Design review of the part built by this model. Coordinates are the model's own, in mm. A direction names the side the tool comes from. Give positions to 0.01 mm unless a question says otherwise; leave off trailing zeros. Loops run counter-clockwise (first coordinate to the right, second up) from the corner with the lowest first, then second, coordinate; pieces in that order, holes last. Notation, with made-up numbers: M 65.5,61 L 118.5,61 A15 cw 118.5,78 Z; hole C -19,56.5 d10. An arc over 180 degrees is marked long. Use CSV: the item, a comma, the result in double quotes.
from build123d import *

# Parameters (mm, degrees)
RESSALTO_EXTRUS_O2_DEPTH  = 19
ESBO_O2_R                 = 2
RESSALTO_EXTRUS_O3_DEPTH  = 5
FILETE1_R                 = 3
ESBO_O3_R                 = 4
RESSALTO_EXTRUS_O4_DEPTH  = 17
RESSALTO_EXTRUS_O6_START  = 10
ESBO_O4_R                 = 4
RESSALTO_EXTRUS_O6_DEPTH  = 10
ESBO_O5_R                 = 4
RESSALTO_EXTRUS_O7_DEPTH  = 10
RESSALTO_EXTRUS_O10_DEPTH = 27
FILETE2_R                 = 10
ESBO_O8_R                 = 5
ESBO_O8_R_2               = 4
RESSALTO_EXTRUS_O11_DEPTH = 2


with BuildPart() as part:
    # Esbo_o1 → Ressalto-extrus_o2 (new body)
    with BuildSketch(Plane.XY):
        with BuildLine():
            Line((-5.964101615, -2), (-3.464101615, -2))
            ThreePointArc((-3.464101615, -2), (4, 0), (-3.464101615, 2))
            Line((-3.464101615, 2), (-5.964101615, 2))
            Line((-5.964101615, 2), (-5.964101615, -2))
        make_face()
    extrude(amount=RESSALTO_EXTRUS_O2_DEPTH)

    # Esbo_o2 → Ressalto-extrus_o3 (add)
    with BuildSketch(Plane.XY.offset(19)):
        with BuildLine():
            Line((-20, -5), (-8.660254038, -5))
            ThreePointArc((-8.660254038, -5), (10, 0), (-8.660254038, 5))
            Line((-8.660254038, 5), (-20, 5))
            Line((-20, 5), (-20, -5))
        make_face()
        with Locations((-15, 0)):
            Circle(ESBO_O2_R, mode=Mode.SUBTRACT)
    extrude(amount=RESSALTO_EXTRUS_O3_DEPTH)

    # Filete1
    filete1_edges = [part.edges().sort_by_distance(p)[0] for p in [
        (-20, 5, 21.5),
        (-20, -5, 21.5),
    ]]
    fillet(filete1_edges, radius=FILETE1_R)

    # Esbo_o3 → Ressalto-extrus_o4 (add)
    with BuildSketch(Plane.XY.offset(24)):
        Circle(ESBO_O3_R)
    extrude(amount=RESSALTO_EXTRUS_O4_DEPTH)

    # Esbo_o5 → Ressalto-extrus_o7 (add)
    with BuildSketch(Plane.XY.offset(41)):
        Circle(ESBO_O5_R)
    extrude(amount=RESSALTO_EXTRUS_O7_DEPTH)



with BuildPart() as body_2:
    # Esbo_o4 → Ressalto-extrus_o6 (new body)
    with BuildSketch(Plane.XY.offset(41).offset(RESSALTO_EXTRUS_O6_START)):
        with BuildLine():
            Line((4, -8), (5, -8))
            ThreePointArc((5, -8), (7.121320344, -7.121320344), (8, -5))
            Line((8, -5), (8, 5))
            ThreePointArc((8, 5), (7.121320344, 7.121320344), (5, 8))
            Line((5, 8), (4, 8))
            Line((4, 8), (-4, 8))
            Line((-4, 8), (-12, 8))
            ThreePointArc((-12, 8), (-20, 0), (-12, -8))
            Line((-12, -8), (-4, -8))
            Line((-4, -8), (4, -8))
        make_face()
        with Locations((-12, 0)):
            Circle(ESBO_O4_R, mode=Mode.SUBTRACT)
    extrude(amount=RESSALTO_EXTRUS_O6_DEPTH)


with BuildPart() as part_1:
    add(part.part)

    add(body_2.part)  # Ressalto-extrus_o10 merges body 2
    # Esbo_o7 → Ressalto-extrus_o10 (add)
    with BuildSketch(Plane.XY.offset(24)):
        with BuildLine():
            Line((0, 8), (0, 4))
            ThreePointArc((0, 4), (2.828427125, 2.828427125), (4, 0))
            ThreePointArc((4, 0), (2.828427125, -2.828427125), (0, -4))
            Line((0, -4), (0, -8))
            Line((0, -8), (5, -8))
            ThreePointArc((5, -8), (5.779003589, -7.897093959), (6.504564394, -7.595435606))
            ThreePointArc((6.504564394, -7.595435606), (7.071067812, -7.071067812), (7.595435606, -6.504564394))
            ThreePointArc((7.595435606, -6.504564394), (7.897093959, -5.779003589), (8, -5))
            Line((8, -5), (8, 5))
            ThreePointArc((8, 5), (7.897093959, 5.779003589), (7.595435606, 6.504564394))
            ThreePointArc((7.595435606, 6.504564394), (7.071067812, 7.071067812), (6.504564394, 7.595435606))
            ThreePointArc((6.504564394, 7.595435606), (5.779003589, 7.897093959), (5, 8))
            Line((5, 8), (0, 8))
        make_face()
    extrude(amount=RESSALTO_EXTRUS_O10_DEPTH)

    # Filete2
    # the kernel refuses this fillet: 10 mm, written as the material it adds along each edge
    with BuildSketch(Plane(origin=(0, -4, 14), x_dir=(0, -1, 0), z_dir=(0, 0, 1))) as filete2_piece_1_section:
        with BuildLine():
            CenterArc((6, -9.797958971), FILETE2_R, 101.536959033, 34.04773237)
            ThreePointArc((-1.142857143, -2.799416849), (-0.296719601, -1.511857892), (0, 0))
            Line((0, 0), (4, 0))
        make_face()
    filete2_piece_1 = extrude(amount=47, mode=Mode.PRIVATE)
    filete2_piece_1 = split(filete2_piece_1, bisect_by=Plane(origin=(-0.997292113, -5.209523734, 19), z_dir=(0, 0, 1)), keep=Keep.TOP, mode=Mode.PRIVATE)
    add(filete2_piece_1)
    with BuildSketch(Plane(origin=(0, 4, 14), x_dir=(-0.9258200997725515, -0.3779644730092269, 0), z_dir=(0, 0, 1))) as filete2_piece_2_section:
        with BuildLine():
            CenterArc((6.803360514, -9.258200998), FILETE2_R, 112.207654299, 34.04773237)
            Line((-1.511857892, -3.703280399), (0, 0))
            ThreePointArc((0, 0), (1.511857892, -0.296719601), (3.023715784, 0))
        make_face()
    filete2_piece_2 = extrude(amount=47, mode=Mode.PRIVATE)
    filete2_piece_2 = split(filete2_piece_2, bisect_by=Plane(origin=(-0.997292113, 5.209523734, 19), z_dir=(0, 0, 1)), keep=Keep.TOP, mode=Mode.PRIVATE)
    add(filete2_piece_2)

    # Esbo_o8 → Ressalto-extrus_o11 (add)
    with BuildSketch(Plane.XY.offset(61)):
        with Locations((-12, 0)):
            Circle(ESBO_O8_R)
        with Locations((-12, 0)):
            Circle(ESBO_O8_R_2, mode=Mode.SUBTRACT)
    extrude(amount=RESSALTO_EXTRUS_O11_DEPTH)


solid = part_1.part
(1) Machinability: for faces 1 (the flat face through (8, 0, 42)), 2 (the flat face through (0.4, 8, 46.4)), 3 (the cylindrical face through (-20, 0, 56)), 4 (the flat face through (-13, -5, 21)), which of the approach directions +Z, -Z, +X, -X, +Y, -Y give a long, thin tool a straight path to every point of the face, cutting with its end or side? Answer none if there is none.
A:
face 1,"+Z, +X, +Y, -Y"
face 2,"+Z, +X, -X, +Y"
face 3,"+Z, -X"
face 4,"-Z, -X, -Y"
(2) We need section A-A on y = 0. State the section outline as (x, z) points, then the cut area to 3 significant figures.
A:
outline,"M -20,19 L -17,19 L -17,24 L -20,24 Z; M -20,51 L -16,51 L -16,63 L -17,63 L -17,61 L -20,61 Z; M -13,19 L -5.96,19 L -5.96,0 L 4,0 L 4,19 L 10,19 L 10,24 L 8,24 L 8,61 L -7,61 L -7,63 L -8,63 L -8,51 L -4,51 L -4,24 L -13,24 Z"
area,"847 mm²"
(3) We need section B-B on z = 29. State the section outline as (x, y) points, then the cut area to 3 significant figures.
A:
outline,"M -2.8,-2.86 A10 cw 0,-8 L 5,-8 A3 ccw 6.5,-7.6 A10 ccw 7.6,-6.5 A3 ccw 8,-5 L 8,5 A3 ccw 7.6,6.5 A10 ccw 6.5,7.6 A3 ccw 5,8 L 0,8 A10 cw -2.8,2.86 A4 ccw Z"
area,"156 mm²"
(4) Wall thickness on line 1 along Y through (x, z) = (-12, 57.5); line 2 along Z through (x, y) = (-4.5, -7.25); line 3 along Y through (x, z) = (-15, 20.25): over which ranges is each line inside the solid? List them lowest first. Write a range as [from, to].
A:
line 1,"[-8, -4], [4, 8]"
line 2,"[19, 24], [51, 61]"
line 3,"[-5, -2], [2, 5]"
(5) We need section D-D on z = 13.5. State the section outline as (x, y) points, then the cut area to 3 significant figures.
A:
outline,"M -5.96,-2 L -3.46,-2 A4 ccw long -3.46,2 L -5.96,2 Z"
area,"58.8 mm²"
(6) The part is to be moulded in two halves that separate along Z. For faces 5 (the flat face through (-3, 0, 61)), 6 (the cylindrical face through (-4, 0, 37)), 7 (the flat face through (-5, -2, 9)), 8 (the cylindrical face through (-1.035, 5.183, 37.311)), say which applies: released by +Z, released by -Z, zero draft, split by the parting line, or undercut.
A:
face 5,"released by +Z"
face 6,"undercut"
face 7,"zero draft"
face 8,"undercut"
(7) We need section C-C on x = -15. State the section outline as (y, z) points, then the cut area to 3 significant figures.
A:
outline,"M -7.42,51 L -2.65,51 L -2.65,63 L -4,63 L -4,61 L -7.42,61 Z; M -5,19 L -2,19 L -2,24 L -5,24 Z; M 2,19 L 5,19 L 5,24 L 2,24 Z; M 2.65,51 L 7.42,51 L 7.42,61 L 4,61 L 4,63 L 2.65,63 Z"
area,"131 mm²"
(8) Clearance check with flat-ended pins moving along their axes: P1, Ø3, axis at x = -6, y = 2.5, coming from the -Z side; P2, Ø0.5, axis at x = 7, y = 7, coming from the -Z side; P3, Ø8, axis at y = 2.5, z = 35.5, coming from the +X side; P4, Ø3, axis at x = -15, y = 0, coming from the -Z side. State where each tip first meets the part, or that it passes through.
A:
P1,"z = 0"
P2,"z = 19"
P3,"x = 8"
P4,"z = 51"
